CAD build for the part. Positions are in the model's coordinates, mm. Face numbers are marked on the shaded views. A direction names the side the tool comes from. Give positions to 0.01 mm unless a question says otherwise; leave off trailing zeros. Write each loop counter-clockwise with the first axis right and the second up, starting at its lowest first coordinate (ties: lowest second). Pieces come first, ordered by that corner, then holes. Notation, with made-up numbers: (78, 64.25) - (106, 64.25) arc R14 cw to (106, 77.25) - close; hole circle Ø9 at (73.5, 31.5). An arc over 180 degrees is marked (long way). Answer as a JSON object with one key per item and string values.
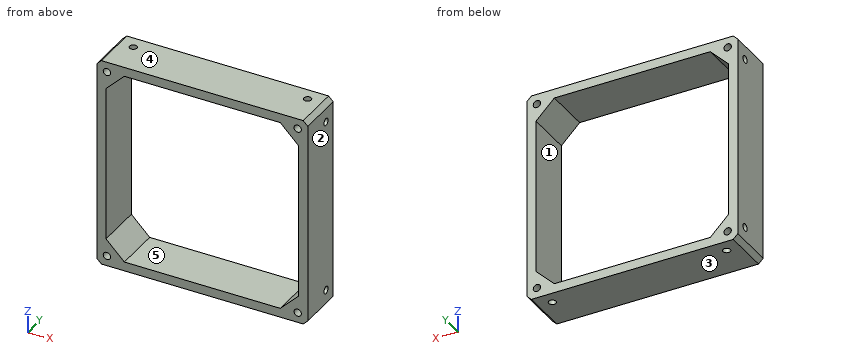
Autodesk Fusion 360 part; units mm, degrees
sketch "Sketch1" plane through (0, 0, 0) normal (0, 1, 0) x (1, 0, 0)
  line L0 (0, 0) -> (46, 0)
  line L1 (46, 0) -> (46, -46)
  line L2 (46, -46) -> (0, -46)
  line L3 (0, -46) -> (0, 0)
  line L4 (0, 0) -> (6.364, -6.364)
  line L5 (0, 0) -> (9, 0) construction
  line L6 (6.364, -6.364) -> (0, -6.364)
  line L7 (0, -6.364) -> (0, 0)
  line L8 (0, 0) -> (6.364, 0)
  line L9 (6.364, 0) -> (6.364, -6.364)
  line L10 (46, -46) -> (37, -46)
  line L11 (37, -46) -> (37, -37)
  line L12 (37, -37) -> (46, -37)
  line L13 (46, -37) -> (46, -46)
  line L14 (46, 0) -> (37, 0)
  line L15 (37, 0) -> (37, -9)
  line L16 (37, -9) -> (46, -9)
  line L17 (46, -9) -> (46, 0)
  line L18 (0, -46) -> (9, -46)
  line L19 (9, -46) -> (9, -37)
  line L20 (9, -37) -> (0, -37)
  line L21 (0, -37) -> (0, -46)
  line L22 (0, -46) -> (2, -46)
  line L23 (2, -46) -> (2, -44)
  circle A0 centre (2, -44) radius 1
  circle A1 centre (2, -44) radius 0.8
  line L24 (23, 0) -> (23, -46)
  line L25 (23, -23) -> (42, -23)
  line L26 (42, -23) -> (42, -42)
  line L27 (42, -42) -> (4, -42)
  line L28 (4, -42) -> (4, -4)
  line L29 (4, -4) -> (42, -4)
  line L30 (42, -4) -> (42, -42)
  line L31 (4, -42) -> (8, -46)
  line L32 (4, -42) -> (9.6569, -42) construction
  line L33 (8, -46) -> (0, -38)
  line L34 (46, -46) -> (44, -46)
  line L35 (44, -46) -> (44, -44)
  circle A2 centre (44, -44) radius 0.8
  line L36 (42, -42) -> (46, -38)
  line L37 (42, -42) -> (38, -46)
  line L38 (46, 0) -> (44, 0)
  line L39 (44, 0) -> (44, -2)
  circle A3 centre (44, -2) radius 0.8
  line L40 (42, -4) -> (46, -8)
  line L41 (46, -8) -> (38, 0)
  line L42 (4, -4) -> (8, 0)
  line L43 (4, -4) -> (0, -8)
  line L44 (0, 0) -> (1.4142, -1.4142)
  circle A4 centre (1.4142, -1.4142) radius 0.8
  line L45 (23, 0) -> (23, -2)
  line L46 (40, -2) -> (6, -2)
  line L47 (44, -6) -> (44, -40)
  line L48 (40, -44) -> (6, -44)
  line L49 (2, -40) -> (2, -6)
  dimension "d1" = 46
  dimension "d2" = 46
  dimension "d3" = 45
  dimension "d4" = 9
  dimension "d5" = 9
  dimension "d6" = 9
  dimension "d7" = 9
  dimension "d8" = 9
  dimension "d9" = 9
  dimension "d10" = 2
  dimension "d11" = 1.6
  dimension "d12" = 19
  dimension "d13" = 19
  dimension "d14" = 45
  dimension "d15" = 1.6
extrude "Extrude1" add sketch "Sketch1" along normal blind 10 contours L3 L4 L6 L7 L43 L44 A4 | L0 L4 L8 L9 L42 L44 A4 | L0 L9 L42 | L3 L6 L43 | L0 L9 L24 L42 L45 L46 | L9 L42 L46 | L3 L6 L20 L43 L49 | L0 L15 L24 L45 L46 | L3 L20 L21 L33 L49 | L0 L14 L15 L41 L46 | L2 L3 L18 L21 L22 L31 L33 | L0 L1 L14 L17 L38 L40 L41 | L2 L18 L19 L31 L33 L48 | L1 L16 L17 L40 L41 L47 | L2 L11 L24 L48 | L2 L19 L24 L48 | L1 L12 L16 L47 | L2 L10 L11 L37 L48 | L1 L2 L10 L13 L34 L36 L37 | L1 L12 L13 L36 L47
sketch "Sketch2" plane through (46, 0, 0) normal (1, 0, 0) x (0, 0, -1)
  line L0 (-46, 0) -> (0, 0)
  line L1 (0, 0) -> (0, 10)
  line L2 (0, 10) -> (-46, 10)
  line L3 (-46, 10) -> (-46, 0)
  line L4 (-43, 0) -> (-43, 7.15)
  line L5 (-43, 7.15) -> (-46.6287, 7.15)
  line L6 (-46, 7.15) -> (-42, 7.15)
  circle A0 centre (-42, 7.15) radius 0.8
extrude "Extrude2" cut sketch "Sketch2" against normal blind 3 contours A0
sketch "Sketch3" plane through (0, 0, 46) normal (0, 0, 1) x (1, 0, 0)
  line L0 (0, 0) -> (46, 0)
  line L1 (46, 0) -> (46, 10)
  line L2 (46, 10) -> (0, 10)
  line L3 (0, 10) -> (0, 0)
  line L4 (43.2, 0) -> (43.2, 7.15)
  line L5 (43.2, 7.15) -> (46.5827, 7.15)
  line L6 (46, 7.15) -> (42, 7.15)
  circle A0 centre (42, 7.15) radius 0.8
  dimension "d20" = 7.15
  dimension "d21" = 1.6
extrude "Extrude3" cut sketch "Sketch3" against normal blind 3 contours A0
sketch "Sketch4" plane through (46, 0, 0) normal (1, 0, 0) x (0, 0, -1)
  circle A0 centre (-42, 7.15) radius 0.8
  line L0 (-46, 0) -> (0, 0)
  line L1 (0, 0) -> (0, 10)
  line L2 (0, 10) -> (-46, 10)
  line L3 (-46, 10) -> (-46, 0)
  line L4 (0, 0) -> (-4, 0)
  line L5 (-4, 0) -> (-4, 7.15)
  circle A1 centre (-4, 7.15) radius 0.8
extrude "Extrude4" cut sketch "Sketch4" against normal blind 3 contours A1
sketch "Sketch5" plane through (0, 0, 0) normal (0, 0, -1) x (-1, 0, 0)
  line L0 (-46, 0) -> (0, 0)
  line L1 (0, 0) -> (0, 10)
  line L2 (0, 10) -> (-46, 10)
  line L3 (-46, 10) -> (-46, 0)
  line L4 (-46, 0) -> (-42, 0)
  line L5 (-42, 0) -> (-42, 7.15)
  circle A0 centre (-42, 7.15) radius 0.8
extrude "Extrude5" cut sketch "Sketch5" against normal blind 3 contours A0
sketch "Sketch6" plane through (0, 0, 0) normal (0, 0, -1) x (-1, 0, 0)
  circle A0 centre (-42, 7.15) radius 0.8
  line L0 (-46, 0) -> (0, 0)
  line L1 (0, 0) -> (0, 10)
  line L2 (0, 10) -> (-46, 10)
  line L3 (-46, 10) -> (-46, 0)
  line L4 (0, 0) -> (-4, 0)
  line L5 (-4, 0) -> (-4, 7.15)
  circle A1 centre (-4, 7.15) radius 0.8
extrude "Extrude6" cut sketch "Sketch6" against normal blind 3 contours A1
sketch "Sketch7" plane through (0, 0, 0) normal (-1, 0, 0) x (0, 0, 1)
  line L0 (0, 0) -> (46, 0)
  line L1 (46, 0) -> (46, 10)
  line L2 (46, 10) -> (0, 10)
  line L3 (0, 10) -> (0, 0)
  line L4 (0, 0) -> (4, 0)
  line L5 (4, 0) -> (4, 7.15)
  line L6 (46, 0) -> (42, 0)
  line L7 (42, 0) -> (42, 7.15)
  circle A0 centre (42, 7.15) radius 0.8
  circle A1 centre (4, 7.15) radius 0.8
extrude "Extrude7" cut sketch "Sketch7" against normal blind 3 contours A1 | A0
sketch "Sketch8" plane through (0, 10, 0) normal (0, 1, 0) x (-1, 0, 0)
  circle A0 centre (-1.4142, 1.4142) radius 0.8
  circle A1 centre (-44, 2) radius 0.8
  line L0 (-44, 40) -> (-42, 42)
  line L1 (-42, 42) -> (-40, 44)
  line L2 (-40, 44) -> (-6, 44)
  line L3 (-6, 44) -> (-2, 40)
  line L4 (-2, 40) -> (-2, 6.364)
  line L5 (-2, 6.364) -> (-1.636, 6.364)
  line L6 (-1.636, 6.364) -> (-6, 2)
  line L7 (-6, 2) -> (-40, 2)
  line L8 (-40, 2) -> (-44, 6)
  line L9 (-44, 6) -> (-44, 40)
  circle A2 centre (-44, 44) radius 0.8
  circle A3 centre (-2, 44) radius 1
  line L10 (-46, 46) -> (-46, 0)
  line L11 (-46, 0) -> (0, 0)
  line L12 (0, 0) -> (0, 46)
  line L13 (0, 46) -> (-46, 46)
  circle A4 centre (-2, 44) radius 1
  circle A5 centre (-2, 44) radius 0.8
extrude "Extrude8" add sketch "Sketch8" against normal blind 10 contours A3 A4
sketch "Sketch9" plane through (0, 0, 46) normal (0, 0, 1) x (1, 0, 0)
  circle A0 centre (42, 7.15) radius 0.8
  line L0 (0, 0) -> (46, 0)
  line L1 (46, 0) -> (46, 10)
  line L2 (46, 10) -> (0, 10)
  line L3 (0, 10) -> (0, 0)
  line L4 (0, 0) -> (4, 0)
  line L5 (4, 0) -> (4, 7.15)
  circle A1 centre (4, 7.15) radius 0.8
extrude "Extrude9" cut sketch "Sketch9" against normal blind 3 contours A1
sketch "Sketch10" plane through (0, 10, 0) normal (0, 1, 0) x (-1, 0, 0)
  circle A0 centre (-2, 44) radius 0.8
  circle A1 centre (-1.4142, 1.4142) radius 0.8
  circle A2 centre (-44, 2) radius 0.8
  line L0 (-44, 40) -> (-42, 42)
  line L1 (-42, 42) -> (-40, 44)
  line L2 (-40, 44) -> (-6, 44)
  line L3 (-6, 44) -> (-2, 40)
  line L4 (-2, 40) -> (-2, 6.364)
  line L5 (-2, 6.364) -> (-1.636, 6.364)
  line L6 (-1.636, 6.364) -> (-6, 2)
  line L7 (-6, 2) -> (-40, 2)
  line L8 (-40, 2) -> (-44, 6)
  line L9 (-44, 6) -> (-44, 40)
  circle A3 centre (-44, 44) radius 0.8
  line L10 (-46, 46) -> (-46, 0)
  line L11 (-46, 0) -> (0, 0)
  line L12 (0, 0) -> (0, 46)
  line L13 (0, 46) -> (-46, 46)
  line L14 (-2, 6.364) -> (-2, 5.5)
  line L15 (-2, 5.5) -> (-1.568, 5.932)
  line L16 (-1.568, 5.932) -> (-1.5, 7)
  line L17 (-1.5, 7) -> (-2, 6.364)
extrude "Extrude10" add sketch "Sketch10" against normal blind 10 contours L5 L6 L14
sketch "Sketch11" plane through (0, 10, 0) normal (0, 1, 0) x (-1, 0, 0)
  circle A0 centre (-2, 44) radius 0.8
  circle A1 centre (-1.4142, 1.4142) radius 0.8
  circle A2 centre (-44, 2) radius 0.8
  line L0 (-44, 40) -> (-42, 42)
  line L1 (-42, 42) -> (-40, 44)
  line L2 (-40, 44) -> (-6, 44)
  line L3 (-6, 44) -> (-2, 40)
  line L4 (-2, 40) -> (-2, 6)
  line L5 (-2, 6) -> (-6, 2)
  line L6 (-6, 2) -> (-40, 2)
  line L7 (-40, 2) -> (-44, 6)
  line L8 (-44, 6) -> (-44, 40)
  circle A3 centre (-44, 44) radius 0.8
  line L9 (-46, 46) -> (-46, 0)
  line L10 (-46, 0) -> (0, 0)
  line L11 (0, 0) -> (0, 46)
  line L12 (0, 46) -> (-46, 46)
  circle A4 centre (-1.4142, 1.4142) radius 0.8
extrude "Extrude11" add sketch "Sketch11" against normal blind 10 contours A1 A4
sketch "Sketch12" plane through (0, 10, 0) normal (0, 1, 0) x (-1, 0, 0)
  circle A0 centre (-2, 44) radius 0.8
  circle A1 centre (-44, 2) radius 0.8
  line L0 (-44, 40) -> (-42, 42)
  line L1 (-42, 42) -> (-40, 44)
  line L2 (-40, 44) -> (-6, 44)
  line L3 (-6, 44) -> (-2, 40)
  line L4 (-2, 40) -> (-2, 6)
  line L5 (-2, 6) -> (-6, 2)
  line L6 (-6, 2) -> (-40, 2)
  line L7 (-40, 2) -> (-44, 6)
  line L8 (-44, 6) -> (-44, 40)
  circle A2 centre (-44, 44) radius 0.8
  line L9 (-46, 46) -> (-46, 0)
  line L10 (-46, 0) -> (0, 0)
  line L11 (0, 0) -> (0, 46)
  line L12 (0, 46) -> (-46, 46)
  line L13 (0, 0) -> (-2, 0)
  line L14 (-2, 0) -> (-2, 2)
  circle A3 centre (-2, 2) radius 0.8
extrude "Extrude12" cut sketch "Sketch12" against normal blind 24.5 contours A3
chamfer "Chamfer1" distance 1 angle 45 4 edges at (0, 5, 0) (0, 5, 46) (46, 5, 46) (46, 5, 0)
sketch "Sketch13" plane through (0, 10, 0) normal (0, 1, 0) x (-1, 0, 0)
  line L0 (-46, 1) -> (-45, 0)
  line L1 (-45, 0) -> (-1, 0)
  line L2 (-1, 0) -> (0, 1)
  line L3 (0, 1) -> (0, 45)
  line L4 (0, 45) -> (-1, 46)
  line L5 (-1, 46) -> (-45, 46)
  line L6 (-45, 46) -> (-46, 45)
  line L7 (-46, 45) -> (-46, 1)
  circle A0 centre (-2, 2) radius 0.8
  circle A1 centre (-2, 44) radius 0.8
  circle A2 centre (-44, 2) radius 0.8
  line L8 (-44, 40) -> (-42, 42)
  line L9 (-42, 42) -> (-40, 44)
  line L10 (-40, 44) -> (-6, 44)
  line L11 (-6, 44) -> (-2, 40)
  line L12 (-2, 40) -> (-2, 6)
  line L13 (-2, 6) -> (-6, 2)
  line L14 (-6, 2) -> (-40, 2)
  line L15 (-40, 2) -> (-44, 6)
  line L16 (-44, 6) -> (-44, 40)
  circle A3 centre (-44, 44) radius 0.8
extrude "Extrude13" add sketch "Sketch13" against normal blind 10 contours A0 | A1 | A2 | A3
sketch "Sketch14" plane through (0, 10, 0) normal (0, 1, 0) x (-1, 0, 0)
  line L0 (-46, 1) -> (-45, 0)
  line L1 (-45, 0) -> (-1, 0)
  line L2 (-1, 0) -> (0, 1)
  line L3 (0, 1) -> (0, 45)
  line L4 (0, 45) -> (-1, 46)
  line L5 (-1, 46) -> (-45, 46)
  line L6 (-45, 46) -> (-46, 45)
  line L7 (-46, 45) -> (-46, 1)
  line L8 (-44, 40) -> (-42, 42)
  line L9 (-42, 42) -> (-40, 44)
  line L10 (-40, 44) -> (-6, 44)
  line L11 (-6, 44) -> (-2, 40)
  line L12 (-2, 40) -> (-2, 6)
  line L13 (-2, 6) -> (-6, 2)
  line L14 (-6, 2) -> (-40, 2)
  line L15 (-40, 2) -> (-44, 6)
  line L16 (-44, 6) -> (-44, 40)
  line L17 (0, 0) -> (-2.2, 0)
  line L18 (-2.2, 0) -> (-2.2, 2.2)
  line L19 (-46, 0) -> (-46, 2.2)
  line L20 (-46, 2.2) -> (-43.8, 2.2)
  line L21 (-46, 46) -> (-46, 43.8)
  line L22 (-46, 43.8) -> (-43.8, 43.8)
  line L23 (0, 46) -> (-2.2, 46)
  line L24 (-2.2, 46) -> (-2.2, 43.8)
  circle A0 centre (-2.2, 43.8) radius 0.8
  circle A1 centre (-43.8, 43.8) radius 0.8
  circle A2 centre (-43.8, 2.2) radius 0.8
  circle A3 centre (-2.2, 2.2) radius 0.8
  dimension "d46" = 2.2
  dimension "d47" = 1.6
extrude "Extrude14" cut sketch "Sketch14" against normal blind 20 contours A3 | A0 | A1 | A2
Item 1: Cut at D-D (z = 26.5). Give the cut face in (x, y).
Entries:
{"outline": "(0, 0) - (2, 0) - (2, 10) - (0, 10) - close; (44, 0) - (46, 0) - (46, 10) - (44, 10) - close"}
Item 2: Probe line 1 (Y direction, x = 2.1, z = 42); line 2 (X direction, y = 8, z = 14). List the from-to ranges inside material, lowest first. Write a range as from..to.
Entries:
{"line 1": "0..6.35, 7.95..10", "line 2": "0..2, 44..46"}
Item 3: Flat gauge pins, fed straight in: P1, Ø1.3, axis at x = 2.2, z = 43.8, coming from the +Y side; P2, Ø1.4, axis at x = 4, y = 7.15, coming from the -Z side. Where does each tip first touch, or does it go through?
Entries:
{"P1": "through", "P2": "z = 3"}
Item 4: Which spindle directions (+Z, -Z, +X, -X, +Y, -Y) get a long thin tool onto all of the face, cutting with end or side? Do the marked faces 4 and 5. Say none if no direction does.
Entries:
{"face 4": "+Z, +X, -X, +Y, -Y", "face 5": "+Y, -Y"}
Item 5: Cut at B-B (y = 5). Give the cut face in (x, z).
Entries:
{"outline": "(0, 1) - (1, 0) - (45, 0) - (46, 1) - (46, 45) - (45, 46) - (1, 46) - (0, 45) - close; hole circle Ø1.6 at (2.2, 2.2); hole circle Ø1.6 at (2.2, 43.8); hole (2, 6) - (6, 2) - (40, 2) - (44, 6) - (44, 40) - (40, 44) - (6, 44) - (2, 40) - close; hole circle Ø1.6 at (43.8, 2.2); hole circle Ø1.6 at (43.8, 43.8)"}
Item 6: Cut at A-A (z = 4). Give the cut face in (x, y).
Entries:
{"outline": "(0, 0) - (4, 0) - (4, 10) - (0, 10) - (0, 7.95) - (3, 7.95) - (3, 6.35) - (0, 6.35) - close; (42, 0) - (46, 0) - (46, 6.35) - (43, 6.35) - (43, 7.95) - (46, 7.95) - (46, 10) - (42, 10) - close"}
Item 7: Cut at C-C (x = 27.5). Give the cut face in (y, z), and give its area (3 significant figures).
Entries:
{"outline": "(0, 0) - (10, 0) - (10, 2) - (0, 2) - close; (0, 44) - (10, 44) - (10, 46) - (0, 46) - close", "area": "40.0 mm2"}
Item 8: Mould opens along X. For the marked faces 1, 2 and 3 say: +X half, -X half, draft (parallel to the pull), parting line (faces both ways), or undercut.
Entries:
{"face 1": "undercut", "face 2": "+X half", "face 3": "draft"}
